from build123d import *

# Parameters (mm, degrees)
SKETCH_1_R      = 1.7
SKETCH_1_R_2    = 1.65
EXTRUDE_1_DEPTH = 4
EXTRUDE_START   = -16
EXTRUDE_2_DEPTH = 16


with BuildPart() as part:
    # Эскиз1 → Бобышка-Вытянуть1 (new body)
    with BuildSketch(Plane(origin=(0, 0, 0), x_dir=(1, 0, 0), z_dir=(0, 1, 0))):
        with BuildLine():
            Line((-9.899164468, -41.277955038), (-5.860900416, -38.382038285))
            add(Edge.make_bspline(
                [(-9.910314442, 27.829010819), (-20.588879158, -13.776681708), (-5.860900416, -38.382038285)],
                knots=[4.008501268, 4.008501268, 4.008501268, 5.815480813, 5.815480813, 5.815480813], degree=2, weights=[1, 0.618872556, 1]))
            ThreePointArc((-9.910314442, 27.829010819), (-11.606984575, 27.965326889), (-13.308802596, 27.998297108))
            add(Edge.make_bspline(
                [(-13.308802596, 27.998297108), (-14.503698084, 24.018467565), (-15.333061847, 19.433308827)],
                knots=[4.040859142, 4.040859142, 4.040859142, 4.265844637, 4.265844637, 4.265844637], degree=2, weights=[1, 0.993679361, 1]))
            Line((-15.333061847, 19.433308827), (-19.381931407, 20.125663445))
            ThreePointArc((-19.381931407, 20.125663445), (-28.959363457, 13.017768481), (-21.429274281, 3.768599193))
            Line((-21.429274281, 3.768599193), (-16.951090448, 3.411043825))
            add(Edge.make_bspline(
                [(-16.951090448, 3.411043825), (-17.049050673, 0), (-16.951090448, -3.411043825)],
                knots=[4.636515229, 4.636515229, 4.636515229, 4.788262732, 4.788262732, 4.788262732], degree=2, weights=[1, 0.997122968, 1]))
            Line((-16.951090448, -3.411043825), (-21.429274281, -3.768599193))
            ThreePointArc((-21.429274281, -3.768599193), (-28.959363457, -13.017768481), (-19.381931407, -20.125663445))
            Line((-19.381931407, -20.125663445), (-15.333061847, -19.433308827))
            add(Edge.make_bspline(
                [(-15.333061847, -19.433308827), (-14.314023938, -25.067085928), (-12.75383545, -29.753186253)],
                knots=[5.158933324, 5.158933324, 5.158933324, 5.434782065, 5.434782065, 5.434782065], degree=2, weights=[1, 0.990503503, 1]))
            Line((-12.75383545, -29.753186253), (-15.8942706, -31.313606592))
            ThreePointArc((-15.8942706, -31.313606592), (-18.296942807, -39.544856639), (-9.899164468, -41.277955038))
        make_face()
        with Locations(Location((-13.298587158, -36.537567928, 0), (0, 0, 270))):
            Circle(SKETCH_1_R, mode=Mode.SUBTRACT)
        with Locations(Location((-20.772601242, 11.993066919, 0), (0, 0, 270))):
            Circle(SKETCH_1_R_2, mode=Mode.SUBTRACT)
        with Locations(Location((-20.772601242, -11.993066919, 0), (0, 0, 270))):
            Circle(SKETCH_1_R_2, mode=Mode.SUBTRACT)
    extrude(amount=EXTRUDE_1_DEPTH)

    # Эскиз2 → Бобышка-Вытянуть2 (add)
    with BuildSketch(Plane(origin=(0, 4, 0), x_dir=(1, 0, 0), z_dir=(0, 1, 0)).offset(EXTRUDE_START)):
        with BuildLine():
            Line((-5, -49.327554721), (-5, -40.655170705))
            add(Edge.make_bspline(
                [(-10.276192518, 27.867200663), (-28.208103976, -18.227340182), (-5, -40.655170705)],
                knots=[3.896305482, 3.896305482, 3.896305482, 5.943348398, 5.943348398, 5.943348398], degree=2, weights=[1, 0.52036205, 1]))
            ThreePointArc((-10.276192518, 27.867200663), (-8.069315303, 27.562444529), (-5.893652235, 27.083201831))
            add(Edge.make_bspline(
                [(-5.893652235, 27.083201831), (-30.674811567, -38), (0, -38)],
                knots=[3.771865525, 3.771865525, 3.771865525, 6.283185307, 6.283185307, 6.283185307], degree=2, weights=[1, 0.309946191, 1]))
            Line((0, -38), (-1, -39))
            Line((-1, -39), (0, -40))
            Line((0, -40), (-1, -41))
            Line((-1, -41), (0, -42))
            Line((0, -42), (-1, -43))
            Line((-1, -43), (0, -44))
            Line((0, -44), (-1, -45))
            Line((-1, -45), (0, -46))
            Line((0, -46), (-1, -47))
            Line((-1, -47), (0, -48))
            Line((0, -48), (-1, -49))
            Line((-1, -49), (0, -50))
            add(Edge.make_bspline(
                [(-5, -49.327554721), (-2.517635123, -50), (0, -50)],
                knots=[2.974009186, 2.974009186, 2.974009186, 3.141592654, 3.141592654, 3.141592654], degree=2, weights=[1, 0.996491526, 1]))
        make_face()
    extrude(amount=EXTRUDE_2_DEPTH)


solid = part.part
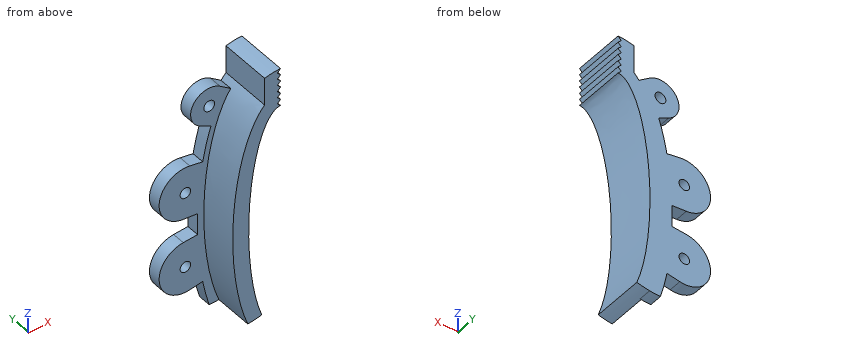
CAD build for the part. Positions are in the model's coordinates, mm. Round coordinates to 2 decimals unless told otherwise and drop trailing zeros. Write each loop counter-clockwise with the first axis right and the second up, starting at its lowest first coordinate (ties: lowest second). Pieces come first, ordered by that corner, then holes.
(1) Probe line 1 along Y through (x, z) = (-18.5, -12); line 2 along Z through (x, y) = (-12.5, 2.25); line 3 along X through (y, z) = (-2.25, 25). List the from-to ranges inside material, lowest first.
(2) Slice it at B-B, the plane x = -24. Write the cut outline in (y, z).
(3) Slice it at A-A, the plane x = -18. Write the cut outline in (y, z).
(4) Drop flat-ended pins along their axis: P1, Ø8, axis at x = -11, y = -10, coming from the +Z side; P2, Ø3, axis at x = -3, y = -8.5, coming from the -Z side; P3, Ø6, axis at y = -6, z = 5.5, coming from the +X side. Give the stop position or say it passes through.
From the geometry:
1. line 1: y = 0 to 4
1. line 2: z = -28 to 35.04, 38.04 to 42.32
1. line 3: x = -12.42 to -7.69
2. outline: (0, -19.59) - (4, -19.59) - (4, -4.4) - (0, -4.4) - close; (0, 4.4) - (4, 4.4) - (4, 19.59) - (0, 19.59) - close
3. outline: (0, -19.89) - (4, -19.89) - (4, -3.49) - (0, -3.49) - close; (0, 3.49) - (4, 3.49) - (4, 19.89) - (0, 19.89) - close; (0, 33.08) - (4, 33.08) - (4, 39.99) - (0, 39.99) - close
4. P1: stops at z = 38.26
4. P2: stops at z = 34.15
4. P3: stops at x = -9.84
